Design review of the part built by this model. Coordinates are the model's own, in mm. A direction names the side the tool comes from. Give positions to 0.01 mm unless a question says otherwise; leave off trailing zeros. Order: outer loops, then holes, each group sorted by start corner. A loop starts at its lowest first (then second) coordinate and runs counter-clockwise, first axis right, second up. Notation, with made-up numbers: M 61.25,-37 L 99.25,-37 A5 cw 99.25,-29 Z; hole C 72,30.25 d9. An arc over 180 degrees is marked long. Answer as a JSON object with one key per item and string values.
from build123d import *

# Parameters (mm, degrees)
F0_W     = 16
F0_H     = 21
F1_DEPTH = 14
F3_DEPTH = 11


with BuildPart() as f1:
    # F0 (on Top) → F1 (new body)
    with BuildSketch(Plane.XY):
        Rectangle(F0_W, F0_H)
    extrude(amount=F1_DEPTH)

    # F2 (on Front) → F3 (cut)
    with BuildSketch(Plane.XZ):
        Polygon((-2, 2), (-2, 1), (2, 1), (2, 2), (3, 2), (3, 4), (6, 4), (6, 11), (-6, 11), (-6, 4), (-3, 4), (-3, 2), align=None)
    extrude(amount=-F3_DEPTH, mode=Mode.SUBTRACT)


solid = f1.part
(1) To check wall thickness, follow L1, parallel to Z at x = 1.75, y = 1; L2, parallel to X at y = 2.25, z = 1.75; L3, parallel to Z at x = -2.25, y = 9.75. State the ranges of each line that lie inside material, in increasing order. Write a range as from..to.
Checked values:
{"L1": "z = 0..1, 11..14", "L2": "x = -8..-2, 2..8", "L3": "z = 0..2, 11..14"}
(2) Draft analysis for pull direction Z (two halves, no side actions). For faces 1 (the flat face through (2.5, 5.2, 2)), 2 (the flat face through (8, 0, 7)), 3 (the flat face through (-3, 5, 3)), 4 (the flat face through (0, 0, 0)), state which applies: +Z half, -Z half, draft (parallel to the pull), parting line (faces both ways), or undercut.
Checked values:
{"face 1": "undercut", "face 2": "draft", "face 3": "undercut", "face 4": "-Z half"}
(3) We need section C-C (z = 8.25). Write out the cut boundary in (x, y), plus the area to 3 significant figures.
Checked values:
{"outline": "M -8,-10.5 L 8,-10.5 L 8,10.5 L 6,10.5 L 6,0 L -6,0 L -6,10.5 L -8,10.5 Z", "area": "210 mm^2"}
(4) We need section B-B (x = 2.5). Write out the cut boundary in (y, z).
Checked values:
{"outline": "M -10.5,0 L 10.5,0 L 10.5,2 L 0,2 L 0,11 L 10.5,11 L 10.5,14 L -10.5,14 Z"}
(5) We need section A-A (y = 6.5). Write out the cut boundary in (x, z), plus the area to 3 significant figures.
Checked values:
{"outline": "M -8,0 L 8,0 L 8,14 L -8,14 Z; hole M -6,4 L -3,4 L -3,2 L -2,2 L -2,1 L 2,1 L 2,2 L 3,2 L 3,4 L 6,4 L 6,11 L -6,11 Z", "area": "124 mm^2"}
(6) Tool access review of faces 5 (the flat face through (-2.5, 5.2, 2)), 6 (the flat face through (0, 0, 14)): name each direction out of +Z, -Z, +X, -X, +Y, -Y from which nothing blocks a thin tool from reaching the whole face with its end or side.
Checked values:
{"face 5": "+Y", "face 6": "+Z, +X, -X, +Y, -Y"}
